```python
from build123d import *

# Parameters (mm, degrees)
SKETCH010_R             = 9
PAD006_DEPTH            = 3
PAD007_DEPTH            = 3
SKETCH012_W             = 2
SKETCH012_H             = 6
PAD008_DEPTH            = 1.5
SKETCH013_W             = 4
SKETCH013_H             = 3
PAD009_DEPTH            = 1.5
BODY004_PLACEMENT_ANGLE = 180


with BuildPart() as part:
    # Sketch010 → Pad006 (new body)
    with BuildSketch(Plane.XZ):
        Polygon((68, 38.5), (68, -38.5), (-3, -38.5), (-3, 38.5), (6.5, 38.5), (6.5, 23), (27.2, 23), (27.2, 38.5), align=None)
        with Locations((23.5, 0)):
            Circle(SKETCH010_R, mode=Mode.SUBTRACT)
    extrude(amount=PAD006_DEPTH)

    # Sketch011 → Pad007 (join)
    with BuildSketch(Plane.XY.offset(24)):
        Polygon((61, 0), (61, 4), (62, 5.5), (61, 7), (59, 7), (59, 0), align=None)
        Polygon((4, 0), (4, 4), (3, 5.5), (4, 7), (6, 7), (6, 0), align=None)
    pad007 = extrude(amount=-PAD007_DEPTH)

    # Mirrored002: Pad007 across XY
    add(pad007.mirror(Plane.XY))

    # Sketch012 → Pad008 (join, symmetric)
    with BuildSketch(Plane.XY):
        with Locations((1, 3)):
            Rectangle(SKETCH012_W, SKETCH012_H)
        with Locations((64, 3)):
            Rectangle(SKETCH012_W, SKETCH012_H)
    extrude(amount=PAD008_DEPTH, both=True)

    # Sketch013 → Pad009 (join, symmetric)
    with BuildSketch(Plane.YZ.offset(34)):
        with Locations((2, -34)):
            Rectangle(SKETCH013_W, SKETCH013_H)
        with Locations((2, 34)):
            Rectangle(SKETCH013_W, SKETCH013_H)
    extrude(amount=PAD009_DEPTH, both=True)


with BuildPart() as part_1:
    # Body004 placement: moved
    add(part.part.moved(Location((0, 55, 0))).rotate(Axis((0, 55, 0), (0, 0, 1)), BODY004_PLACEMENT_ANGLE))


solid = part_1.part
```
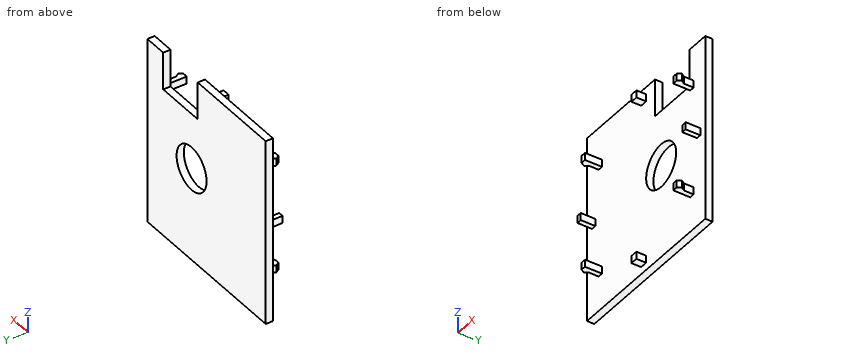
CAD build for the part. Positions are in the model's coordinates, mm. Round coordinates to 2 decimals unless told otherwise and drop trailing zeros. Loops run counter-clockwise (first coordinate to the right, second up) from the corner with the lowest first, then second, coordinate; pieces in that order, holes last. Notation, with made-up numbers: (-37.75, -28.5) - (9.25, -28.5) arc R18 ccw to (9.25, -19.5) - close; hole circle Ø6 at (-39, 15.25). An arc over 180 degrees is marked (long way). Return JSON: item names as keys, results as strings. Group by question number.
Q1. Drill centre lines: line 1 along Z through (x, y) = (-23.5, 56.2); line 2 along Y through (x, z) = (-29.5, 23); line 3 along Z through (x, y) = (-4.5, 51.5). Where is each one in solid material? Low to high. Write a range as [from, to].
Q2. Band-saw the part on B-B on x = -23.5. Give the cut face in (y, z).
Q3. Band-saw the part on D-D on z = 0. Give the cut face in (x, y).
Q4. Band-saw the part on C-C on y = 53.5. Give the number of separate pieces and of enclosed holes in the cut face, plus the area to 3 significant figures.
Q5. Flat gauge pins, fed straight in: pin 1 Ø3.5 at (y, z) = (50.5, -0.5) entering from +X; pin 2 Ø3.5 at (y, z) = (52, -22.5) entering from -X; pin 3 Ø3.5 at (y, z) = (52.5, 0.5) entering from -X. Where does each tip first touch, or does it go through?
Q6. Band-saw the part on A-A on z = 29. Give the cut face in (x, y), plus the area to 3 significant figures.
Solutions:
{
 "1": {"line 1": "z = [-38.5, -9], [9, 23]", "line 2": "y = [55, 58]", "line 3": "z = [-24, -21], [21, 24]"},
 "2": {"outline": "(55, -38.5) - (58, -38.5) - (58, -9) - (55, -9) - close; (55, 9) - (58, 9) - (58, 23) - (55, 23) - close"},
 "3": {"outline": "(-68, 55) - (-65, 55) - (-65, 49) - (-63, 49) - (-63, 55) - (-32.5, 55) - (-32.5, 58) - (-68, 58) - close; (-14.5, 55) - (-2, 55) - (-2, 49) - (0, 49) - (0, 55) - (3, 55) - (3, 58) - (-14.5, 58) - close"},
 "4": {"separate pieces": "8", "enclosed holes": "0", "area": "54.0 mm^2"},
 "5": {"pin 1": "stops at x = 0", "pin 2": "stops at x = -61.5", "pin 3": "stops at x = -65"},
 "6": {"outline": "(-68, 55) - (-27.2, 55) - (-27.2, 58) - (-68, 58) - close; (-6.5, 55) - (3, 55) - (3, 58) - (-6.5, 58) - close", "area": "151 mm^2"}
}
